Could you check a few things on this model? Use its own coordinates, in mm. Face numbers are marked on the shaded views. A direction names the side the tool comes from. Round coordinates to 2 decimals unless told otherwise and drop trailing zeros. Write each loop counter-clockwise with the first axis right and the second up, starting at its lowest first coordinate (ties: lowest second). Pieces come first, ordered by that corner, then holes.
Autodesk Inventor part; units mm, degrees
ref_plane "Work Plane1" through (0, 20, 0) normal (0, 1, 0) x (-1, 0, 0)
ref_plane "YZ Plane" through (0, 0, 0) normal (1, 0, 0) x (0, 1, 0)
ref_plane "XY Plane" through (0, 0, 0) normal (0, 0, 1) x (1, 0, 0)
sketch "Sketch1" plane through (0, 0, 0) normal (0, 0, 1) x (1, 0, 0)
  circle A0 centre (0, 0) radius 14.5
  circle A1 centre (11.5, 0) radius 1.5
  line L0 (0, 16.0858) -> (0, -16.9174) construction
  line L1 (-27.4443, 0) -> (33.7473, 0) construction
  circle A2 centre (-11.5, 0) radius 1.5
  circle A3 centre (0, 0) radius 8.25
  dimension "d0" = 29
  dimension "d1" = 3
  dimension "d2" = 11.5
  dimension "d3" = 16.5
extrude "Extrusion1" add sketch "Sketch1" along normal blind 3
sketch "Sketch2" plane through (0, 0, 0) normal (0, 0, -1) x (-1, 0, 0)
  circle A0 centre (0, 0) radius 9
  dimension "d6" = 18
extrude "Extrusion2" add sketch "Sketch2" along normal blind 31
fillet "Fillet1" radius 2 1 edges at (9, 0, 0)
sketch "Sketch3" plane through (0, 0, 0) normal (0, 0, 1) x (1, 0, 0)
  circle A0 centre (0, 0) radius 8.25
extrude "Extrusion3" cut sketch "Sketch3" against normal blind 30
ref_plane "Work Plane1" through (0, 20, 0) normal (0, 1, 0) x (-1, 0, 0)
sketch "Sketch5" plane through (0, 20, 0) normal (0, 1, 0) x (-1, 0, 0)
  line L0 (-25, -10) -> (25, -10)
  line L1 (25, -10) -> (25, -20)
  line L2 (25, -20) -> (-25, -20)
  line L3 (-25, -20) -> (-25, -10)
  line L4 (-25, -10) -> (25, -20) construction
  line L5 (25, -10) -> (-25, -20) construction
  point P0 (0, 0)
  point P1 (0, -15)
  dimension "d19" = 50
  dimension "d20" = 10
  dimension "d27" = 15
extrude "Extrusion5" add sketch "Sketch5" against normal blind 3
fillet "Fillet3" radius 2 4 edges at (-25, 18.5, -10) (-25, 18.5, -20) (25, 18.5, -10) (25, 18.5, -20)
sketch "Sketch6" plane through (0, 17, 0) normal (0, -1, 0) x (1, 0, 0)
  line L0 (-5, -20) -> (5, -20)
  line L1 (5, -20) -> (5, -10)
  line L2 (5, -10) -> (-5, -10)
  line L3 (-5, -10) -> (-5, -20)
  line L4 (-5, -20) -> (5, -10) construction
  line L5 (5, -20) -> (-5, -10) construction
  point P0 (0, 0)
  point P1 (0, -15)
  dimension "d24" = 10
  dimension "d25" = 10
  dimension "d26" = 15
extrude "Extrusion6" add sketch "Sketch6" along normal up to next
fillet "Fillet4" radius 2 2 edges at (5, 17, -15) (-5, 17, -15)
fillet "Fillet5" radius 2 2 edges at (0, 9, -10) (0, 9, -20)
sketch "Sketch7" plane through (0, 20, 0) normal (0, 1, 0) x (1, 0, 0)
  circle A0 centre (18, 15) radius 3.25
  circle A1 centre (-18, 15) radius 3.25
  line L0 (0, -10.182) -> (0, 25.8871) construction
  line L1 (-23, 10) -> (23, 10)
  point P0 (0, 0)
  dimension "d32" = 6.5
  dimension "d33" = 6.5
  dimension "d34" = 36
  dimension "d35" = 5
extrude "Extrusion7" cut sketch "Sketch7" against normal blind 10
properties part number "AcopleTC"
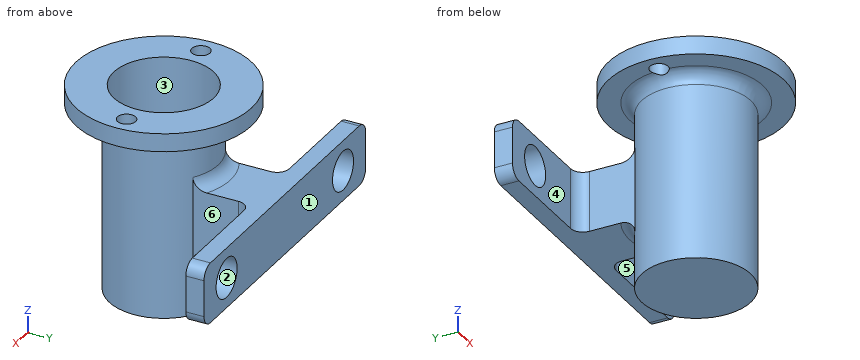
Q1. Imagine slicing it at B-B, the plane y = 0. Write out the boundary of the cut face in (x, z), then the cut area to 3 significant figures.
Q2. We'd pull the mould along Y, two halves only. Please class the marked faces 1, 2 and 3: pulls with the +Y half, pulls with the -Y half, needs draft (parallel to the pull), parting line crosses it, or undercut.
Q3. Imagine slicing it at A-A, the plane x = 18. Write out the boundary of the cut face in (y, z).
Q4. Imagine slicing it at D-D, the plane z = -7. Write out the boundary of the cut face in (x, y).
Q5. On a 3-axis mill with a long thin cutter (end or side, diameter ignored), from which of +Z, -Z, +X, -X, +Y, -Y can I reach the whole of each face in a straight line? I mean the marked faces 4, 5 and 6. Say none if no direction works.
Q6. Imagine slicing it at C-C, the plane x = -11.5. Write out the boundary of the cut face in (y, z).
Q7. If I drill on L1, parallel to X at y = 18.9, z = -15; L2, parallel to Y at x = 0, z = -4; L3, parallel to Z at x = -3, y = 13, over which ranges is the centre line in solid material (lowest first)?
Q8. I'm going to push flat-ended pins straight in: pin 1 Ø8 at (x, z) = (-11.5, -15) entering from -Y; pin 2 Ø5 at (x, y) = (-3, -1) entering from +Z; pin 3 Ø11 at (x, y) = (0.5, 16) entering from -Z. Where does each tip first touch, or does it pass through?
Results found:
1. outline: (-14.5, 0) - (-13, 0) - (-13, 3) - (-14.5, 3) - close; (-10, -0.27) arc R2 cw to (-9, -2) - (-9, -31) - (9, -31) - (9, -2) arc R2 cw to (10, -0.27) - (10, 3) - (8.25, 3) - (8.25, -30) - (-8.25, -30) - (-8.25, 3) - (-10, 3) - close; (13, 0) - (14.5, 0) - (14.5, 3) - (13, 3) - close
1. area: 84.0 mm2
2. face 1: pulls with the +Y half
2. face 2: needs draft
2. face 3: undercut
3. outline: (17, -20) - (20, -20) - (20, -18.25) - (17, -18.25) - close; (17, -11.75) - (20, -11.75) - (20, -10) - (17, -10) - close
4. outline: circle Ø18 at (0, 0); hole circle Ø16.5 at (0, 0)
5. face 4: +Z, -Z, -X
5. face 5: +Z, -Z, +X
5. face 6: -Z, +X
6. outline: (-8.83, 0) - (-1.5, 0) - (-1.5, 3) - (-8.83, 3) - close; (1.5, 0) - (8.83, 0) - (8.83, 3) - (1.5, 3) - close; (17, -20) - (20, -20) - (20, -10) - (17, -10) - close
7. L1: x = -25 to -21.25, -14.75 to 14.75, 21.25 to 25
7. L2: y = -9 to -8.25, 8.25 to 9
7. L3: z = -20 to -10, 0 to 3
8. pin 1: stops at y = -4.97
8. pin 2: stops at z = -30
8. pin 3: stops at z = -20.06
